from build123d import *

# Parameters (mm, degrees)
ESBO_O1_W                                            = 66
ESBO_O1_H                                            = 30
RESSALTO_EXTRUS_O1_DEPTH                             = 5
ESBO_O2_W                                            = 66
ESBO_O2_H                                            = 9
CORTE_EXTRUS_O1_DEPTH                                = 1
FURO_ROSCADO_PARA_CONDU_TE_DE_M2_2X0_451_D           = 2.3
FURO_ROSCADO_PARA_CONDU_TE_DE_M2_2X0_451_DEPTH       = 6
FURO_ROSCADO_PARA_CONDU_TE_DE_M2_2X0_451_CSINK_D     = 2.895
FURO_ROSCADO_PARA_CONDU_TE_DE_M2_2X0_451_CSINK_ANGLE = 90
FURO_ROSCADO_PARA_CONDU_TE_DE_M2_2X0_451_TIP         = 0.690989712
FURO_ROSCADO_PARA_CONDU_TE_DE_M2_2X0_452_D           = 2.3
FURO_ROSCADO_PARA_CONDU_TE_DE_M2_2X0_452_DEPTH       = 6
FURO_ROSCADO_PARA_CONDU_TE_DE_M2_2X0_452_CSINK_D     = 2.895
FURO_ROSCADO_PARA_CONDU_TE_DE_M2_2X0_452_CSINK_ANGLE = 90
FURO_ROSCADO_PARA_CONDU_TE_DE_M2_2X0_452_TIP         = 0.690989712
FURO_ROSCADO_PARA_CONDU_TE_DE_M3X0_53_D              = 3.15
FURO_ROSCADO_PARA_CONDU_TE_DE_M3X0_53_CSINK_D        = 3.766
FURO_ROSCADO_PARA_CONDU_TE_DE_M3X0_53_CSINK_ANGLE    = 90


with BuildPart() as part:
    # Esboço1 → Ressalto-extrusão1 (new body)
    with BuildSketch(Plane(origin=(0, 0, 0), x_dir=(1, 0, 0), z_dir=(0, 1, 0))):
        Rectangle(ESBO_O1_W, ESBO_O1_H)
    extrude(amount=RESSALTO_EXTRUS_O1_DEPTH)

    # Esboço2 → Corte-extrusão1 (cut)
    with BuildSketch(Plane(origin=(0, 5, 0), x_dir=(1, 0, 0), z_dir=(0, 1, 0))):
        Rectangle(ESBO_O2_W, ESBO_O2_H)
    extrude(amount=-CORTE_EXTRUS_O1_DEPTH, mode=Mode.SUBTRACT)

    # Furo roscado para conduíte de M2.2x0.451
    with Locations(Plane(origin=(33, 0, 0), x_dir=(0, 0, -1), z_dir=(1, 0, 0))):
        with Locations((-10, 2.5), (10, 2.5)):
            CounterSinkHole(FURO_ROSCADO_PARA_CONDU_TE_DE_M2_2X0_451_D / 2, FURO_ROSCADO_PARA_CONDU_TE_DE_M2_2X0_451_CSINK_D / 2, depth=FURO_ROSCADO_PARA_CONDU_TE_DE_M2_2X0_451_DEPTH, counter_sink_angle=FURO_ROSCADO_PARA_CONDU_TE_DE_M2_2X0_451_CSINK_ANGLE)
            with Locations((0, 0, -(FURO_ROSCADO_PARA_CONDU_TE_DE_M2_2X0_451_DEPTH + FURO_ROSCADO_PARA_CONDU_TE_DE_M2_2X0_451_TIP / 2))):  # 118° drill point
                Cone(0, FURO_ROSCADO_PARA_CONDU_TE_DE_M2_2X0_451_D / 2, FURO_ROSCADO_PARA_CONDU_TE_DE_M2_2X0_451_TIP, mode=Mode.SUBTRACT)

    # Furo roscado para conduíte de M2.2x0.452
    with Locations(Plane.ZY.offset(33)):
        with Locations((-10, 2.5), (10, 2.5)):
            CounterSinkHole(FURO_ROSCADO_PARA_CONDU_TE_DE_M2_2X0_452_D / 2, FURO_ROSCADO_PARA_CONDU_TE_DE_M2_2X0_452_CSINK_D / 2, depth=FURO_ROSCADO_PARA_CONDU_TE_DE_M2_2X0_452_DEPTH, counter_sink_angle=FURO_ROSCADO_PARA_CONDU_TE_DE_M2_2X0_452_CSINK_ANGLE)
            with Locations((0, 0, -(FURO_ROSCADO_PARA_CONDU_TE_DE_M2_2X0_452_DEPTH + FURO_ROSCADO_PARA_CONDU_TE_DE_M2_2X0_452_TIP / 2))):  # 118° drill point
                Cone(0, FURO_ROSCADO_PARA_CONDU_TE_DE_M2_2X0_452_D / 2, FURO_ROSCADO_PARA_CONDU_TE_DE_M2_2X0_452_TIP, mode=Mode.SUBTRACT)

    # Furo roscado para conduíte de M3x0.53 (through all)
    with Locations(Plane(origin=(0, 4, 0), x_dir=(1, 0, 0), z_dir=(0, 1, 0))):
        with Locations((-21, 0), (-1, 0), (19, 0)):
            CounterSinkHole(FURO_ROSCADO_PARA_CONDU_TE_DE_M3X0_53_D / 2, FURO_ROSCADO_PARA_CONDU_TE_DE_M3X0_53_CSINK_D / 2, counter_sink_angle=FURO_ROSCADO_PARA_CONDU_TE_DE_M3X0_53_CSINK_ANGLE)


solid = part.part
Here's how the part is built. I have some questions about the finished solid (model axes, mm). A direction names the side the tool comes from. Round coordinates to 2 decimals unless told otherwise and drop trailing zeros. Order: outer loops, then holes, each group sorted by start corner. A loop starts at its lowest first (then second) coordinate and runs counter-clockwise, first axis right, second up. Notation, with made-up numbers: (59, 24) -> (81, 24) arc R4 cw to (81, 30) -> close; hole circle Ø6 at (-8.75, 36.25). An arc over 180 degrees is marked (long way). Use CSV: the item, a comma, the result in double quotes.
1. I want a section at B-B on z = 0. List the corners of the cut face in (x, y) for me (3 decimals).
Recorded:
outline,"(-33, 0) -> (-22.575, 0) -> (-22.575, 3.692) -> (-22.883, 4) -> (-33, 4) -> close; (-19.425, 0) -> (-2.575, 0) -> (-2.575, 3.692) -> (-2.883, 4) -> (-19.117, 4) -> (-19.425, 3.692) -> close; (0.575, 0) -> (17.425, 0) -> (17.425, 3.692) -> (17.117, 4) -> (0.883, 4) -> (0.575, 3.692) -> close; (20.575, 0) -> (33, 0) -> (33, 4) -> (20.883, 4) -> (20.575, 3.692) -> close"
2. I want a section at A-A on x = 19. List the corners of the cut face in (y, z) for me (3 decimals), and give its area (3 significant figures).
Recorded:
outline,"(0, -15) -> (5, -15) -> (5, -4.5) -> (4, -4.5) -> (4, -1.883) -> (3.692, -1.575) -> (0, -1.575) -> close; (0, 1.575) -> (3.692, 1.575) -> (4, 1.883) -> (4, 4.5) -> (5, 4.5) -> (5, 15) -> (0, 15) -> close"
area,"128 mm2"
3. Which directions (+Z, -Z, +X, -X, +Y, -Y) give clear straight access to the entire face, cutting with the end or side of a thin tool? Please do faces 4 (the face through (0, 2, -15)), 5 (the face through (29.811, 2.06, 11.062)).
Recorded:
face 4,"-Z, +X, -X, +Y, -Y"
face 5,"+X"
4. I'm going to push flat-ended pins straight in: P1, Ø1.4, axis at y = 2.5, z = 10, coming from the -X side; P2, Ø1.8, axis at y = 2.5, z = -10, coming from the -X side; P3, Ø1.9, axis at x = -1, z = 0, coming from the +Y side; P4, Ø1, axis at x = 15.5, z = -3.5, coming from the +Y side. Where does each tip first touch, or does it pass through?
Recorded:
P1,"stops at x = -26.73"
P2,"stops at x = -26.85"
P3,"passes through"
P4,"stops at y = 4"
5. I need wall thicknesses on line 1 along Z through (x, y) = (29.25, 2.5); line 2 along Y through (x, z) = (-30.85, 10); line 3 along Z through (x, y) = (-10, 4.4). Which ranges of each line are inside material? Lowest first, please.
Recorded:
line 1,"z = -15 to -11.15, -8.85 to 8.85, 11.15 to 15"
line 2,"y = 0 to 1.35, 3.65 to 5"
line 3,"z = -15 to -4.5, 4.5 to 15"
6. I want a section at C-C on x = 12. List the corners of the cut face in (y, z) for me, and give its area (3 significant figures).
Recorded:
outline,"(0, -15) -> (5, -15) -> (5, -4.5) -> (4, -4.5) -> (4, 4.5) -> (5, 4.5) -> (5, 15) -> (0, 15) -> close"
area,"141 mm2"
7. Thinking about a two-plate mould opening in X: for faces 1 (the face through (-33, 2, 0)), 2 (the face through (-29.811, 2.06, -11.062)), 3 (the face through (17.498, 1.82, -0.473)), which applies, pulls with the +X half, pulls with the -X half, needs draft (parallel to the pull), parting line crosses it, or undercut?
Recorded:
face 1,"pulls with the -X half"
face 2,"needs draft"
face 3,"undercut"
